The drawing under review shows one solid part. Ordinate dimensions are in mm from its lowest x, y, z. Round coordinates to 2 decimals unless told otherwise and drop trailing zeros. Order: outer loops, then holes, each group sorted by start corner. A loop starts at its lowest first (then second) coordinate and runs counter-clockwise, first axis right, second up.
1) Consider section B-B (x = 21). Give the boundary of the cut face in (y, z), then the cut area to 3 significant figures.
2) Clearance check with flat-ended pins moving along their axes: P1, Ø3, axis at y = 42, z = 2, coming from the +X side; P2, Ø1.5, axis at x = 11.5, z = 2, coming from the -Y side; P3, Ø3, axis at y = 39.5, z = 2.5, coming from the -X side. State where each tip first meets the part, or that it passes through.
3) To check wall thickness, follow L1, parallel to Y at x = 52, z = 0.75; L2, parallel to Y at x = 36.5, z = 4.05; L3, parallel to X at y = 42, z = 1.05. State the ranges of each line that lie inside material, in increasing order.
4) Consider section A-A (z = 1.15). Give the boundary of the cut face in (x, y).
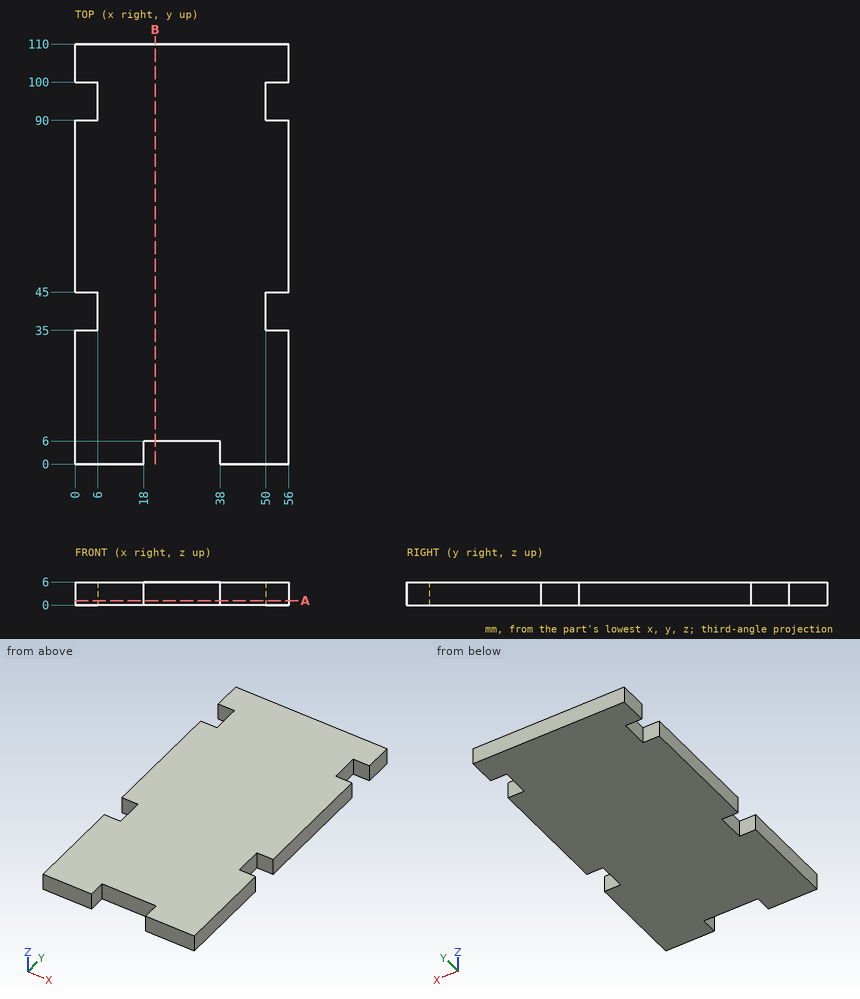
Answer below:
1. outline: (6, 0) - (110, 0) - (110, 6) - (6, 6) - close
1. area: 624 mm2
2. P1: stops at x = 50
2. P2: stops at y = 0
2. P3: stops at x = 6
3. L1: y = 0 to 35, 45 to 90, 100 to 110
3. L2: y = 6 to 110
3. L3: x = 6 to 50
4. outline: (0, 0) - (18, 0) - (18, 6) - (38, 6) - (38, 0) - (56, 0) - (56, 35) - (50, 35) - (50, 45) - (56, 45) - (56, 90) - (50, 90) - (50, 100) - (56, 100) - (56, 110) - (0, 110) - (0, 100) - (6, 100) - (6, 90) - (0, 90) - (0, 45) - (6, 45) - (6, 35) - (0, 35) - close
